Verification items for the finished model (mm, model axes). Give positions to 0.01 mm unless a question says otherwise; leave off trailing zeros. Order: outer loops, then holes, each group sorted by start corner. A loop starts at its lowest first (then second) coordinate and runs counter-clockwise, first axis right, second up.
(1) Scan lines: L1, parallel to Z at x = 0, y = 2; L2, parallel to Z at x = -10, y = 1.7; L3, parallel to X at y = 0.7, z = -46. Record each from-to range of solid material in increasing order.
(2) Sectioned sample at D-D on z = -42.5. Record the cut outline in (x, y).
(3) Sectioned sample at C-C on x = 10. Record the cut outline in (y, z), plus the area to 4 significant figures.
(4) Sectioned sample at A-A on x = -45. Record the cut outline in (y, z), plus the area to 3 significant figures.
(5) Gauge pin test, flat ends, axial feed: pin 1 (0.9 mm diameter, centred on x = -4, y = 1.5, fed in from +Z); pin 2 (8 mm diameter, centred on x = -45.5, z = -51.5, fed in from +Y). Record the tip position at first contact, or that the pin passes through.
(6) Sectioned sample at B-B on y = 2.3. Count the separate pieces of the cut face and the enclosed holes in it, plus the area to 3 significant figures.
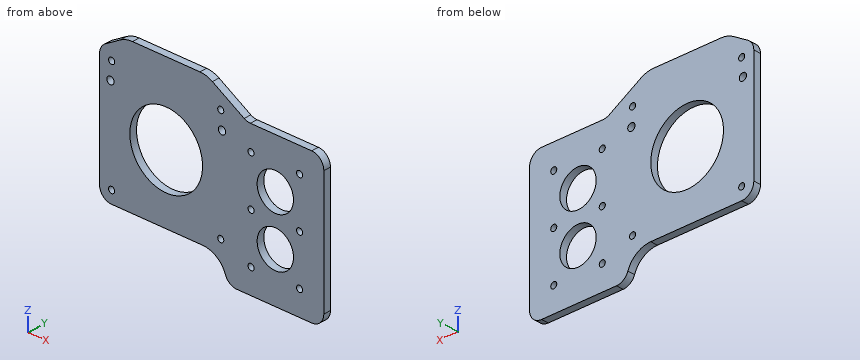
Autodesk Inventor part; units mm, degrees
ref_plane "YZ Plane" through (0, 0, 0) normal (1, 0, 0) x (0, 1, 0)
ref_plane "XZ Plane" through (0, 0, 0) normal (0, 1, 0) x (-1, 0, 0)
ref_plane "XY Plane" through (0, 0, 0) normal (0, 0, 1) x (1, 0, 0)
sketch "Sketch1" plane through (0, 0, 0) normal (0, 1, 0) x (-1, 0, 0)
  line L0 (10, 0) -> (80, 0)
  line L1 (90, -32.6619) -> (90, -167.3381)
  line L2 (67, -200) -> (23, -200)
  line L3 (0, -167.3381) -> (0, -85)
  line L4 (68, -27) -> (68, -173) construction
  line L5 (68, -173) -> (22, -173) construction
  line L6 (22, -173) -> (22, -27) construction
  circle A0 centre (68, -27) radius 1.5
  circle A1 centre (68, -173) radius 1.5
  circle A2 centre (22, -173) radius 1.5
  circle A3 centre (22, -27) radius 1.5
  line L7 (30, -70) -> (60, -70)
  line L8 (70, -80) -> (70, -120)
  line L9 (60, -130) -> (30, -130)
  line L10 (20, -120) -> (20, -80)
  arc A4 (70, -80) -> (60, -70) centre (60, -80) ccw
  arc A5 (60, -130) -> (70, -120) centre (60, -120) ccw
  arc A6 (20, -120) -> (30, -130) centre (30, -120) ccw
  arc A7 (30, -70) -> (20.5719, -76.6667) centre (30, -80) ccw
  arc A8 (90, -10) -> (80, 0) centre (80, -10) ccw
  arc A9 (0, -190) -> (10, -200) centre (10, -190) ccw
  arc A10 (80, -200) -> (90, -190) centre (80, -190) ccw
  arc A11 (10, 0) -> (0, -10) centre (10, -10) ccw
  circle A12 centre (80, -10) radius 1.25
  circle A13 centre (80, -30) radius 1.25
  circle A14 centre (80, -50) radius 1.25
  circle A15 centre (80, -70) radius 1.25
  circle A16 centre (80, -90) radius 1.25
  circle A17 centre (80, -110) radius 1.25
  circle A18 centre (80, -130) radius 1.25
  circle A19 centre (80, -150) radius 1.25
  circle A20 centre (80, -170) radius 1.25
  circle A21 centre (80, -190) radius 1.25
  circle A22 centre (10, -10) radius 1.25
  circle A23 centre (10, -30) radius 1.25
  circle A24 centre (10, -50) radius 1.25
  circle A25 centre (10, -70) radius 1.25
  circle A26 centre (10, -90) radius 1.25
  circle A27 centre (10, -110) radius 1.25
  circle A28 centre (10, -130) radius 1.25
  circle A29 centre (10, -150) radius 1.25
  circle A30 centre (10, -170) radius 1.25
  circle A31 centre (10, -190) radius 1.25
  circle A32 centre (81, -111) radius 3.5
  circle A33 centre (81.25, -89) radius 3.5
  circle A34 centre (9, -111) radius 3.5
  circle A35 centre (9, -89) radius 3.5
  line L11 (70.0725, -15.0435) -> (64.0418, -11.4251)
  line L12 (12.8542, -19.2875) -> (25.9582, -11.4251)
  arc A36 (90, -32.6619) -> (85.145, -24.087) centre (80, -32.6619) ccw
  arc A37 (4.855, -24.087) -> (0, -32.6619) centre (10, -32.6619) ccw construction
  circle A38 centre (67.5, -65) radius 1.25
  circle A39 centre (22.5, -65) radius 1.25
  line L13 (-15, -70) -> (15, -70)
  circle A40 centre (67.5, -20) radius 1.25
  line L14 (30, -25) -> (60, -25)
  circle A41 centre (22.5, -20) radius 1.25
  line L15 (-15, -25) -> (15, -25) construction
  line L16 (58.8968, -10) -> (31.1032, -10)
  arc A42 (64.0418, -11.4251) -> (58.8968, -10) centre (58.8968, -20) ccw
  arc A43 (31.1032, -10) -> (25.9582, -11.4251) centre (31.1032, -20) ccw
  line L17 (90, -200) -> (72, -200) construction
  line L18 (72, -195) -> (72, -185)
  line L19 (77, -180) -> (85, -180)
  line L20 (90, -175) -> (90, -167.3381)
  line L21 (0, -200) -> (18, -200) construction
  line L22 (18, -195) -> (18, -185)
  line L23 (13, -180) -> (5, -180)
  line L24 (0, -175) -> (0, -167.3381)
  arc A44 (77, -180) -> (72, -185) centre (77, -185) ccw
  arc A45 (85, -180) -> (90, -175) centre (85, -175) ccw
  arc A46 (0, -175) -> (5, -180) centre (5, -175) ccw
  arc A47 (18, -185) -> (13, -180) centre (13, -185) ccw
  arc A48 (67, -200) -> (72, -195) centre (67, -195) ccw
  arc A49 (18, -195) -> (23, -200) centre (23, -195) ccw
  circle A50 centre (69.1385, -144.2) radius 1.25
  circle A51 centre (20.8615, -144.2) radius 1.25
  circle A52 centre (53.8985, -195) radius 1.25
  line L25 (10, -30) -> (-10, -30) construction
  line L26 (-10, -30) -> (-10, -50) construction
  line L27 (-10, -50) -> (10, -50) construction
  line L28 (10, -50) -> (10, -30) construction
  circle A53 centre (-10, -50) radius 1.25
  circle A54 centre (-10, -30) radius 1.25
  line L29 (-10, -30) -> (-10, -20) construction
  line L30 (-10, -20) -> (10.2817, -20)
  line L31 (-10, -20) -> (-15, -20)
  line L32 (-20, -25) -> (-20, -75)
  line L33 (-15, -80) -> (-5, -80)
  arc A55 (-15, -20) -> (-20, -25) centre (-15, -25) ccw
  arc A56 (-20, -75) -> (-15, -80) centre (-15, -75) ccw
  arc A57 (0, -85) -> (-5, -80) centre (-5, -85) ccw
  arc A58 (10.2817, -20) -> (12.8542, -19.2875) centre (10.2817, -15) ccw
  line L34 (-10, -50) -> (-10, -70) construction
  circle A59 centre (-10, -70) radius 1.25
  line L35 (-10, -80) -> (15.8579, -80)
  line L36 (60, -70) -> (67.5, -70)
  line L37 (72.5, -65) -> (72.5, -19.331)
  arc A60 (72.5, -19.331) -> (70.0725, -15.0435) centre (67.5, -19.331) ccw
  arc A61 (67.5, -70) -> (72.5, -65) centre (67.5, -65) ccw
  arc A62 (15.8579, -80) -> (20.5719, -76.6667) centre (15.8579, -75) ccw
  line L38 (10, -70) -> (-10, -50) construction
  line L39 (10, -30) -> (-10, -50) construction
  circle A63 centre (0, -60) radius 7.5
  circle A64 centre (0, -40) radius 7.5
  line L40 (67.5, -65) -> (22.5, -20) construction
  circle A65 centre (45, -42.5) radius 15
  point P0 (0, 0)
  point P1 (90, 0)
  point P2 (70, -130)
  point P3 (70, -70)
  point P4 (20, -130)
  point P5 (45, 0)
  point P6 (45, -200)
  point P7 (25, -70)
  point P8 (70, -25)
  point P9 (25, -25)
  point P10 (72, -180)
  point P11 (-20, -20)
  point P12 (-20, -80)
  point P13 (72.5, -70)
  dimension "d0" = 90
  dimension "d1" = 200
  dimension "d2" = 46
  dimension "d4" = 22
  dimension "d5" = 27
  dimension "d7" = 3
  dimension "d8" = 3
  dimension "d10" = 50
  dimension "d11" = 60
  dimension "d12" = 20
  dimension "d13" = 70
  dimension "d14" = 10
  dimension "d15" = 10
  dimension "d16" = 2.5
  dimension "d19" = 20
  dimension "d24" = 2.5
  dimension "d27" = 20
  dimension "d34" = 7
  dimension "d35" = 7
  dimension "d36" = 7
  dimension "d37" = 7
  dimension "d38" = 72
  dimension "d39" = 22
  dimension "d40" = 9
  dimension "d41" = 89
  dimension "d42" = 22
  dimension "d43" = 72
  dimension "d46" = 10
  dimension "d48" = 2.5
  dimension "d51" = 45
  dimension "d54" = 45
  dimension "d57" = 22.5
  dimension "d58" = 5
  dimension "d71" = 18
  dimension "d72" = 20
  dimension "d73" = 18
  dimension "d74" = 5
  dimension "d75" = 5
  dimension "d76" = 2.5
  dimension "d77" = 2.5
  dimension "d78" = 0
  dimension "d79" = 48.277
  dimension "d81" = 20.8615
  dimension "d82" = 2.5
  dimension "d83" = 15.24
  dimension "d84" = 50.8
  dimension "d85" = 5
  dimension "d86" = 20
  dimension "d87" = 20
  dimension "d88" = 2.5
  dimension "d89" = 2.5
  dimension "d92" = 10
  dimension "d93" = 10
  dimension "d94" = 60
  dimension "d95" = 5
  dimension "d96" = 5
  dimension "d97" = 20
  dimension "d98" = 2.5
  dimension "d99" = 12.5
  dimension "d100" = 5
  dimension "d101" = 5
  dimension "d102" = 15
  dimension "d103" = 15
  dimension "d104" = 30
extrude "Extrusion2" add sketch "Sketch1" along normal blind 3 contours A7 A62 L35 L33 A56 L32 A55 L31 L30 A58 L12 A43 L16 A42 L11 A60 L37 A61 L36 L7
equation "\"d4\" = -0.5 * d2 + 0.5 * d0"
equation "\"d5\" = -0.5 * d3 + 0.5 * d1"
equation "\"d12\" = -0.5 * d10 + 0.5 * d0"
equation "\"d13\" = -0.5 * d11 + 0.5 * d1"
equation "\"d40\" = -0.5 * d38 + 0.5 * d0"
equation "\"d41\" = -0.5 * d39 + 0.5 * d1"
equation "\"d57\" = -0.5 * d51 + 0.5 * d0"
equation "\"d81\" = -0.5 * d79 + 0.5 * d0"
properties part number "TransmissionDeck" material "Polycarbonate, Clear"
Ans:
1. L1: z = -80 to -67.5, -52.5 to -47.5, -32.5 to -20
1. L2: z = -80 to -71.25, -68.75 to -51.25, -48.75 to -31.25, -28.75 to -20
1. L3: x = -72.5 to -59.59, -30.41 to -4.5, 4.5 to 20
2. outline: (-72.5, 0) - (-60, 0) - (-60, 3) - (-72.5, 3) - close; (-30, 0) - (-7.07, 0) - (-7.07, 3) - (-30, 3) - close; (7.07, 0) - (20, 0) - (20, 3) - (7.07, 3) - close
3. outline: (0, -80) - (3, -80) - (3, -71.25) - (0, -71.25) - close; (0, -68.75) - (3, -68.75) - (3, -51.25) - (0, -51.25) - close; (0, -48.75) - (3, -48.75) - (3, -31.25) - (0, -31.25) - close; (0, -28.75) - (3, -28.75) - (3, -20) - (0, -20) - close
3. area: 157.5 mm2
4. outline: (0, -70) - (3, -70) - (3, -57.5) - (0, -57.5) - close; (0, -27.5) - (3, -27.5) - (3, -10) - (0, -10) - close
4. area: 90.0 mm2
5. pin 1: stops at z = -20
5. pin 2: passes through
6. separate pieces: 1
6. enclosed holes: 15
6. area: 4,390 mm2
